Check sheet for the modelled part. Datum: model origin and axes. Units: mm. A direction names the side the tool comes from. Give positions to 0.01 mm unless a question says otherwise; leave off trailing zeros. Loops run counter-clockwise (first coordinate to the right, second up) from the corner with the lowest first, then second, coordinate; pieces in that order, holes last. Notation, with made-up numbers: M -9.5,-1 L 19.5,-1 A9 ccw 19.5,3 Z; hole C 19.5,54 d7. An arc over 180 degrees is marked long. Write each question's results on one line, items separated by ' | '. Start each with the question number.
1. Sectioned sample at C-C on y = -79. Record the cut outline in (x, z) (3 decimals).
2. Tool access check on faces 1 (the flat face through (-19.05, -63, -1)), 2 (the cylindrical face through (-4.87, -118.75, -15.17)), 3 (the cylindrical face through (-6.71, 15.17, -0.62)). Record the directions out of +Z, -Z, +X, -X, +Y, -Y that give a thin tool (end or side, any length) a straight path to the whole face; none if there is none.
3. Sectioned sample at A-A on x = -11.43. Record the cut outline in (y, z) (1 decimal).
4. Material ranges on line 1 along Z through (x, y) = (-5.5, -8.5) (3 decimals); line 2 along X through (y, z) = (-98.5, 1); line 3 along Y through (x, z) = (-19, -6), recorded low to high.
5. Go/stop test with flat-tipped pins: pin 1 (2 mm diameter, centred on x = -9, y = -89, fed in from -Z) (3 decimals); pin 2 (2.5 mm diameter, centred on x = -21, z = -4, fed in from -Y); pin 3 (13.5 mm diameter, centred on y = -94.5, z = 2, fed in from +X); pin 4 (12 mm diameter, centred on y = -57.5, z = -18.5, fed in from +X). Record where each tip stops, or that it passes through.
6. Draft check along X on faces 4 (the flat face through (-26.67, 5, -1)), 5 (the flat face through (-5, -123, -24.765)), 6 (the cylindrical face through (2.86, 15.17, -1.74)). Enter one of: pulls with the +X half, pulls with the -X half, needs draft (parallel to the pull), parting line crosses it, or undercut.
7. Sectioned sample at D-D on x = 1.27. Record the cut outline in (y, z) (3 decimals).
8. Sectioned sample at B-B on z = 0. Record the cut outline in (x, y).
```python
from build123d import *

# Parameters (mm, degrees)
SKETCH1_W              = 33.02
SKETCH1_H              = 19.05
BOSS_EXTRUDE1_DEPTH    = 10.16
SKETCH2_R              = 4.7625
SKETCH2_R_2            = 2.357295936
BOSS_EXTRUDE2_DEPTH    = 10.16
SKETCH5_W              = 19.05
SKETCH5_H              = 10.16
BOSS_EXTRUDE3_DEPTH    = 5.08
SKETCH6_W              = 19.05
SKETCH6_H              = 10.16
BOSS_EXTRUDE4_DEPTH    = 5.08
SKETCH7_W              = 27.94
SKETCH7_H              = 19.05
BOSS_EXTRUDE5_DEPTH    = 128.27
SKETCH9_R              = 4.7625
BOSS_EXTRUDE6_DEPTH    = 15.24
CUT_EXTRUDE3_START     = -21.717
CUT_EXTRUDE3_OUTLINE_R = 4.7625
CUT_EXTRUDE3_DEPTH     = 0.7366
SKETCH13_R             = 4.4704
BOSS_EXTRUDE8_DEPTH    = 0.7366
SKETCH14_W             = 27.94
SKETCH14_H             = 10.16
CUT_EXTRUDE4_DEPTH     = 15.24
SKETCH15_W             = 43.18
SKETCH15_H             = 138.43
CUT_EXTRUDE5_DEPTH     = 2.032


# Read off the part's stored shape, not the designer's step: Cut-Extrude3
with BuildPart() as part:
    # Sketch1 → Boss-Extrude1 (new body)
    with BuildSketch(Plane(origin=(0, 0, 0), x_dir=(1, 0, 0), z_dir=(0, 1, 0))):
        with Locations((-5.08, 0)):
            Rectangle(SKETCH1_W, SKETCH1_H)
    extrude(amount=BOSS_EXTRUDE1_DEPTH)

    # Sketch2 → Boss-Extrude2 (add)
    with BuildSketch(Plane(origin=(0, 10.16, 0), x_dir=(1, 0, 0), z_dir=(0, 1, 0))):
        with Locations(Location((-11.43, 0, 0), (0, 0, 270))):
            Circle(SKETCH2_R)
        with Locations(Location((1.27, 0, 0), (0, 0, 270))):
            Circle(SKETCH2_R_2)
    extrude(amount=BOSS_EXTRUDE2_DEPTH)

    # Sketch5 → Boss-Extrude3 (add)
    with BuildSketch(Plane.ZY.offset(21.59)):
        with Locations((0, 5.08)):
            Rectangle(SKETCH5_W, SKETCH5_H)
    extrude(amount=BOSS_EXTRUDE3_DEPTH)

    # Sketch6 → Boss-Extrude4 (add)
    with BuildSketch(Plane(origin=(11.43, 0, 0), x_dir=(0, 0, -1), z_dir=(1, 0, 0))):
        with Locations((0, 5.08)):
            Rectangle(SKETCH6_W, SKETCH6_H)
    extrude(amount=BOSS_EXTRUDE4_DEPTH)

    # Sketch7 → Boss-Extrude5 (add)
    with BuildSketch(Plane(origin=(0, 0, 0), x_dir=(-1, 0, 0), z_dir=(0, -1, 0))):
        with Locations((5.08, 0)):
            Rectangle(SKETCH7_W, SKETCH7_H)
    extrude(amount=BOSS_EXTRUDE5_DEPTH)

    # Sketch9 → Boss-Extrude6 (add)
    with BuildSketch(Plane.XY.offset(9.525)):
        with Locations(Location((-5.08, -123.5075, 0), (0, 0, 270))):
            Circle(SKETCH9_R)
    boss_extrude6 = extrude(amount=BOSS_EXTRUDE6_DEPTH)

    # Mirror5: Boss-Extrude6 across plane
    add(boss_extrude6.mirror(Plane.XY))

    # Cut-Extrude3 outline → Cut-Extrude3 (cut)
    with BuildSketch(Plane.XY.offset(CUT_EXTRUDE3_START)):
        with Locations((-5.08, -123.5075)):
            Circle(CUT_EXTRUDE3_OUTLINE_R)
    extrude(amount=CUT_EXTRUDE3_DEPTH, mode=Mode.SUBTRACT)

    # Sketch13 → Boss-Extrude8 (add)
    with BuildSketch(Plane(origin=(0, 0, -20.9804), x_dir=(-1, 0, 0), z_dir=(0, 0, -1))):
        with Locations(Location((5.08, -123.5075, 0), (0, 0, 180))):
            Circle(SKETCH13_R)
    extrude(amount=BOSS_EXTRUDE8_DEPTH)

    # Sketch14 → Cut-Extrude4 (cut)
    with BuildSketch(Plane.XY.offset(9.525)):
        with Locations((-5.08, -123.19)):
            Rectangle(SKETCH14_W, SKETCH14_H)
    extrude(amount=CUT_EXTRUDE4_DEPTH, mode=Mode.SUBTRACT)

    # Sketch15 → Cut-Extrude5 (cut)
    with BuildSketch(Plane.XY.offset(9.525)):
        with Locations((-5.08, -59.055)):
            Rectangle(SKETCH15_W, SKETCH15_H)
    extrude(amount=-CUT_EXTRUDE5_DEPTH, mode=Mode.SUBTRACT)


solid = part.part
```
Output values:
1) outline: M -19.05,-9.525 L 8.89,-9.525 L 8.89,7.493 L -19.05,7.493 Z
2) face 1: +Z, -Z, -X, -Y | face 2: -Z | face 3: +Y
3) outline: M -128.3,-9.5 L 10.2,-9.5 L 10.2,-4.8 L 20.3,-4.8 L 20.3,4.8 L 10.2,4.8 L 10.2,7.5 L -128.3,7.5 Z
4) line 1: -9.525 to 7.493 | line 2: -19.05 to 8.89 | line 3: -128.27 to 10.16
5) pin 1: z = -9.525 | pin 2: y = 0 | pin 3: x = 8.89 | pin 4: through
6) face 4: pulls with the -X half | face 5: needs draft | face 6: undercut
7) outline: M -128.27,-9.525 L 10.16,-9.525 L 10.16,-2.357 L 20.32,-2.357 L 20.32,2.357 L 10.16,2.357 L 10.16,7.493 L -128.27,7.493 Z
8) outline: M -26.67,0 L -19.05,0 L -19.05,-128.27 L 8.89,-128.27 L 8.89,0 L 16.51,0 L 16.51,10.16 L 3.63,10.16 L 3.63,20.32 L -1.09,20.32 L -1.09,10.16 L -6.67,10.16 L -6.67,20.32 L -16.19,20.32 L -16.19,10.16 L -26.67,10.16 Z
